Geometry check sheet. Reference: the model listing, model coordinates, mm. Face numbers are marked on the shaded views. A direction names the side the tool comes from. Round coordinates to 2 decimals unless told otherwise and drop trailing zeros. Loops run counter-clockwise (first coordinate to the right, second up) from the corner with the lowest first, then second, coordinate; pieces in that order, holes last. Notation, with made-up numbers: (-1, 70.5) - (49, 70.5) arc R27 cw to (49, 86.5) - close; hole circle Ø11 at (77, -31). An arc over 180 degrees is marked (long way). Write item = value, one per line.
```python
from build123d import *

# Parameters (mm, degrees)
SKETCH1_W           = 44
SKETCH1_H           = 44
SKETCH1_R           = 2
SKETCH1_R_2         = 10
BOSS_EXTRUDE1_DEPTH = 10
SKETCH2_R           = 18
SKETCH2_R_2         = 10
BOSS_EXTRUDE2_DEPTH = 27
FILLET1_R           = 5


with BuildPart() as part:
    # Sketch1 → Boss-Extrude1 (new body)
    with BuildSketch(Plane(origin=(0, 0, 0), x_dir=(0, 0, -1), z_dir=(1, 0, 0))):
        Rectangle(SKETCH1_W, SKETCH1_H)
        with Locations((-15.556349186, 15.556349186)):
            Circle(SKETCH1_R, mode=Mode.SUBTRACT)
        with Locations((15.556349186, 15.556349186)):
            Circle(SKETCH1_R, mode=Mode.SUBTRACT)
        with Locations((15.556349186, -15.556349186)):
            Circle(SKETCH1_R, mode=Mode.SUBTRACT)
        with Locations((-15.556349186, -15.556349186)):
            Circle(SKETCH1_R, mode=Mode.SUBTRACT)
        Circle(SKETCH1_R_2, mode=Mode.SUBTRACT)
    extrude(amount=BOSS_EXTRUDE1_DEPTH)

    # Sketch2 → Boss-Extrude2 (add)
    with BuildSketch(Plane(origin=(0, 0, 0), x_dir=(0, 0, -1), z_dir=(1, 0, 0))):
        Circle(SKETCH2_R)
        Circle(SKETCH2_R_2, mode=Mode.SUBTRACT)
    extrude(amount=BOSS_EXTRUDE2_DEPTH)

    # Fillet1
    fillet1_edges = [part.edges().sort_by_distance(p)[0] for p in [
        (5, 22, 22),
        (5, 22, -22),
        (5, -22, -22),
        (5, -22, 22),
    ]]
    fillet(fillet1_edges, radius=FILLET1_R)


solid = part.part
```
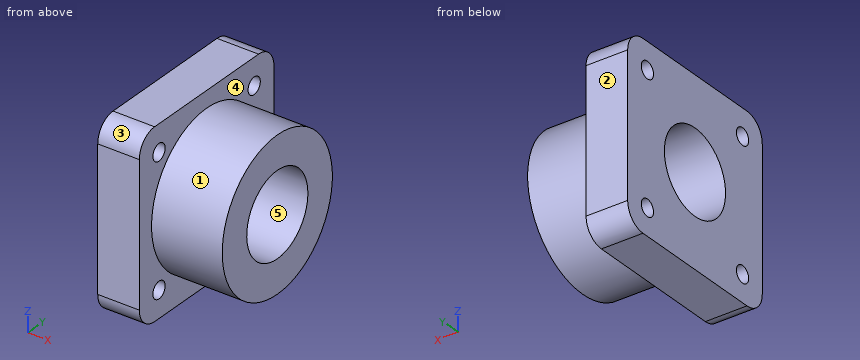
(1) Gauge pin test, flat ends, axial feed: pin 1 (3 mm diameter, centred on x = 21, y = 6, fed in from -Z); pin 2 (5 mm diameter, centred on x = 16, z = -12, fed in from +Y). Record the tip position at first contact, or that the pin passes through.
Answers follow:
pin_1 = -17.43
pin_2 = 15.29
(2) Mould release check, pull along Z, two halves, no side actions. Record for the marked faces 3, 4 and 5: pulls with the +Z half, pulls with the -Z half, needs draft (parallel to the pull), parting line crosses it, or undercut.
Answers follow:
face_3 = pulls with the +Z half
face_4 = needs draft
face_5 = undercut
(3) Section check D-D (z = 12). Enter the section's corners in (x, y).
Answers follow:
outline = (0, -22) - (10, -22) - (10, -13.42) - (27, -13.42) - (27, 13.42) - (10, 13.42) - (10, 22) - (0, 22) - close
(4) Set-up check for the marked faces 1 and 2: record each of +Z, -Z, +X, -X, +Y, -Y from which the full face is reachable in a straight line by a thin tool's end or side.
Answers follow:
face_1 = +X
face_2 = +Z, -Z, +X, -X, +Y
(5) Scan lines: L1, parallel to Z at x = 5.5, y = -15.5; L2, parallel to Y at x = 7.5, z = 15; L3, parallel to Y at x = 5, z = 17. Record each from-to range of solid material in increasing order. Write a range as [from, to].
Answers follow:
L1 = [-22, -17.56], [-13.56, 13.56], [17.56, 22]
L2 = [-22, -17.48], [-13.64, 13.64], [17.48, 22]
L3 = [-22, -16.94], [-14.17, 14.17], [16.94, 22]
(6) Section check A-A (z = 0). Enter the section's corners in (x, y), then the cut area to 3 significant figures.
Answers follow:
outline = (0, -22) - (10, -22) - (10, -18) - (27, -18) - (27, -10) - (0, -10) - close; (0, 10) - (27, 10) - (27, 18) - (10, 18) - (10, 22) - (0, 22) - close
area = 512 mm²
(7) Section check C-C (x = 22). Enter the section's corners in (y, z).
Answers follow:
outline = circle Ø36 at (0, 0); hole circle Ø20 at (0, 0)
